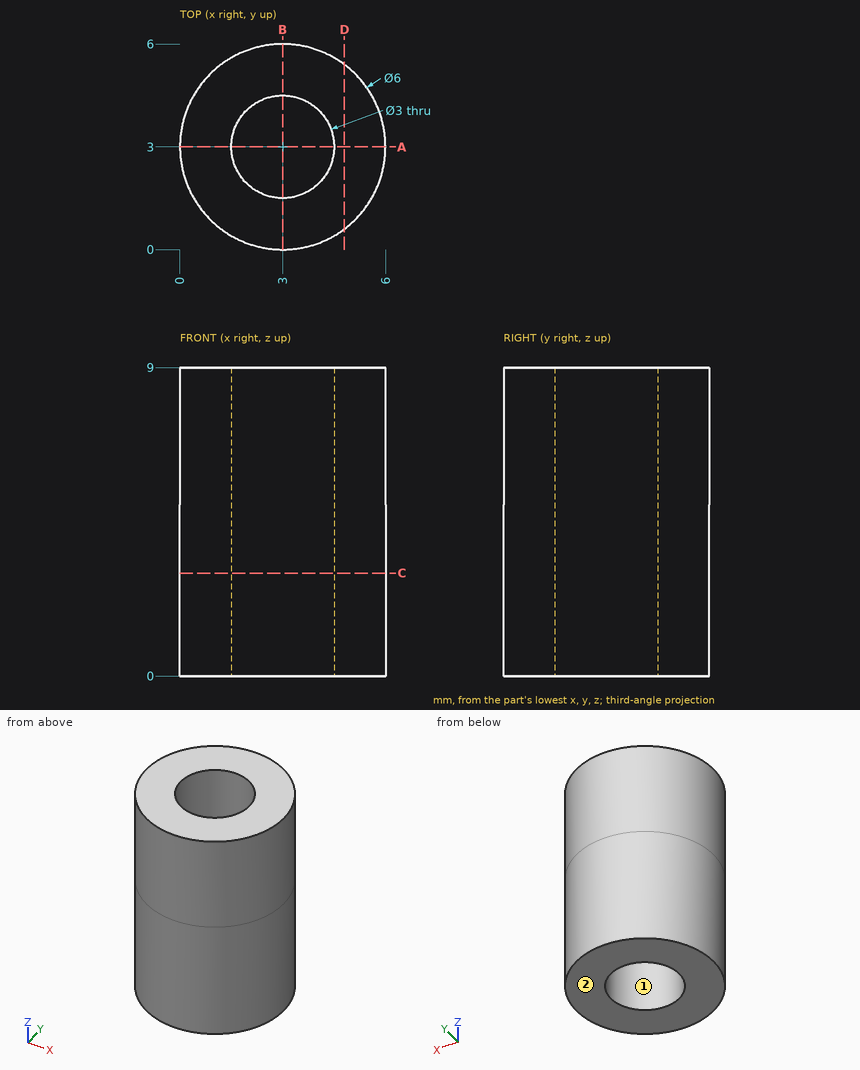
Answer from the drawing. Dimensions are ordinates in mm from the lowest x, y and z of the part. Coordinates: 2 decimals unless noted, no trailing zeros. Write each loop counter-clockwise with the first axis right and the second up, starting at its lowest first coordinate (ties: lowest second). Pieces come first, ordered by that corner, then holes. Notation, with made-up numbers: M -7,1.25 L 44,1.25 A34 ccw 44,35.25 Z; hole C 14,77 d2. An arc over 180 degrees is marked long. Use a Markdown table: item, result.
Q1. Straight lines are drawn through the part: L1, parallel to Y at x = 3, z = 2.25; L2, parallel to X at y = 4.25, z = 5.5; L3, parallel to X at y = 2.4, z = 4.5. For each, find the intervals that lie inside material, in ascending order. Write a range as [from, to].
Answer block:
| item | result |
|---|---|
| L1 | y = [0, 1.5], [4.5, 6] |
| L2 | x = [0.27, 2.17], [3.83, 5.73] |
| L3 | x = [0.06, 1.63], [4.37, 5.94] |
Q2. The part is cut by section A-A, the plane y = 3. Write down the section's boundary in (x, z).
Answer block:
| item | result |
|---|---|
| outline | M 0,0 L 1.5,0 L 1.5,9 L 0,9 Z; M 4.5,0 L 6,0 L 6,9 L 4.5,9 Z |
Q3. Each of these flat-tipped pins is pushed along its axis until it touches: pin 1 Ø1 at (x, z) = (2, 2) entering from -Y; pin 2 Ø1.5 at (y, z) = (4, 8) entering from +X; pin 3 Ø1 at (y, z) = (2, 2.5) entering from -X. Where does it stop, or does it pass through?
Answer block:
| item | result |
|---|---|
| pin 1 | stops at y = 0.04 |
| pin 2 | stops at x = 5.99 |
| pin 3 | stops at x = 0.04 |
Q4. Determine the mould class of the marked faces 1 and 2 for opening direction X: released by +X, released by -X, zero draft, split by the parting line, or undercut.
Answer block:
| item | result |
|---|---|
| face 1 | undercut |
| face 2 | zero draft |
Q5. The part is cut by section C-C, the plane z = 3. Write down the section's boundary in (x, y).
Answer block:
| item | result |
|---|---|
| outline | C 3,3 d6; hole C 3,3 d3 |
Q6. The part is cut by section D-D, the plane x = 4.8. Write down the section's boundary in (y, z).
Answer block:
| item | result |
|---|---|
| outline | M 0.6,0 L 5.4,0 L 5.4,9 L 0.6,9 Z |
